Can you work these out from the model? Positions are in its coordinate system, mm. Face numbers are marked on the shaded views. A direction names the side the tool comes from. Give positions to 0.01 mm unless a question says otherwise; leave off trailing zeros. Order: outer loops, then holes, each group sorted by start corner. A loop starts at its lowest first (then second) coordinate and runs counter-clockwise, first axis right, second up. Notation, with made-up numbers: M 86.25,38 L 103.25,38 A25 ccw 103.25,70 Z; hole C 31,5 d3. An arc over 180 degrees is marked long. Write each question's results on one line, items separated by ' | '.
from build123d import *

# Parameters (mm, degrees)
SKETCH1_R           = 9
SKETCH1_R_2         = 7
BOSS_EXTRUDE1_DEPTH = 10
FILLET1_R           = 1
SKETCH2_W           = 18
SKETCH2_H           = 18
BOSS_EXTRUDE2_DEPTH = 10
CUT_EXTRUDE1_DEPTH  = 23.472205054


with BuildPart() as part:
    # Sketch1 → Boss-Extrude1 (new body)
    with BuildSketch(Plane(origin=(0, 0, 0), x_dir=(1, 0, 0), z_dir=(0, 1, 0))):
        with Locations(Location((0, 0, 0), (0, 0, 270))):
            Circle(SKETCH1_R)
        with Locations(Location((0, 0, 0), (0, 0, 270))):
            Circle(SKETCH1_R_2, mode=Mode.SUBTRACT)
    extrude(amount=BOSS_EXTRUDE1_DEPTH)

    # Fillet1
    fillet1_edges = [part.edges().sort_by_distance(p)[0] for p in [
        (0, 10, -9),
        (0, 10, -7),
    ]]
    fillet(fillet1_edges, radius=FILLET1_R - 0.0001)  # a hair under: the kernel refuses the full size

    # Sketch2 → Boss-Extrude2 (add)
    with BuildSketch(Plane.XZ):
        Rectangle(SKETCH2_W, SKETCH2_H)
    extrude(amount=BOSS_EXTRUDE2_DEPTH)

    # Sketch4 → Cut-Extrude1 (cut, through all)
    with BuildSketch(Plane.XY.offset(9)):
        Polygon((-9, -10), (9, -10), (9, -1.969771915), align=None)
    extrude(amount=-CUT_EXTRUDE1_DEPTH, mode=Mode.SUBTRACT)


solid = part.part
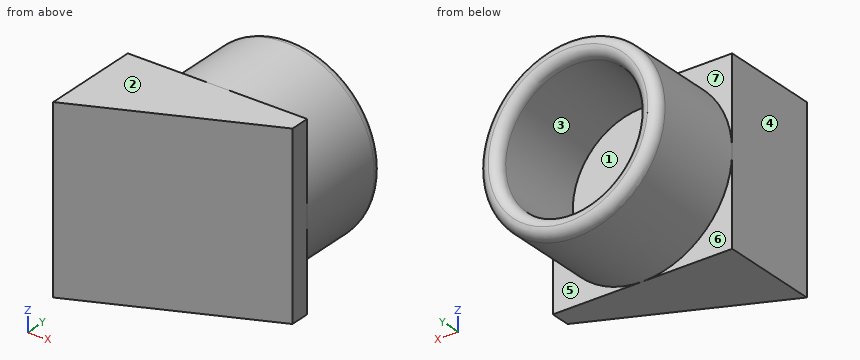
(1) For the marked faces 5, 6 and 7, which set-ups out of +Z, -Z, +X, -X, +Y, -Y let a thin tool reach every point of the face, with its end or its side?
Data:
face 5: -Z, +X, +Y | face 6: -Z, -X, +Y | face 7: +Z, -X, +Y
(2) Will these pins go through, and if not, where does the flat tip stop? P1, Ø2, axis at x = 6, y = 6.5, coming from the -Z side; P2, Ø4, axis at x = 2.5, z = 5, coming from the +Y side; P3, Ø7, axis at x = 1.5, z = 2, coming from the +Y side.
Data:
P1: stops at z = -7.48 | P2: stops at y = 9.91 | P3: stops at y = 0
(3) We'd pull the mould along Z, two halves only. Please class the marked faces 1, 2, 3 and 4: +Z half, -Z half, draft (parallel to the pull), parting line (faces both ways), or undercut.
Data:
face 1: undercut | face 2: +Z half | face 3: undercut | face 4: draft
(4) I need wall thicknesses on L1, parallel to X at y = 4, z = 0; L2, parallel to X at y = 8, z = 5.25; L3, parallel to Z at x = 2.5, y = 6.75. Which ranges of each line are inside material? Lowest first, please. Write a range as from..to.
Data:
L1: x = -9..-7, 7..9 | L2: x = -7.31..-4.63, 4.63..7.31 | L3: z = -8.65..-6.54, 6.54..8.65
(5) Imagine slicing it at A-A, the plane y = 8. Write out the boundary of the cut face in (x, z), plus the area to 3 significant figures.
Data:
outline: C 0,0 d18; hole C 0,0 d14 | area: 101 mm2
(6) Imagine slicing it at C-C, the plane y = -7.25. Write out the boundary of the cut face in (x, z).
Data:
outline: M -9,-9 L -2.84,-9 L -2.84,9 L -9,9 Z
(7) Imagine slicing it at B-B, the plane y = -4. Write out the boundary of the cut face in (x, z), plus the area to 3 significant figures.
Data:
outline: M -9,-9 L 4.45,-9 L 4.45,9 L -9,9 Z | area: 242 mm2
